The listing builds one solid part. Answer for the finished solid, in the listing's coordinates (mm). Face numbers are marked on the shaded views. A direction names the side the tool comes from. Give positions to 0.01 mm unless a question says otherwise; leave off trailing zeros. Write each loop counter-clockwise with the first axis right and the second up, starting at its lowest first coordinate (ties: lowest second). Pieces come first, ordered by that corner, then holes. Notation, with made-up numbers: (-8.5, 24.25) -> (-3.5, 24.25) arc R17 cw to (-3.5, 31.25) -> close; hole circle Ø4 at (85, 62.25). An arc over 180 degrees is marked (long way). Use CSV: the item, a comma, the result in double quotes. Start each with the question number.
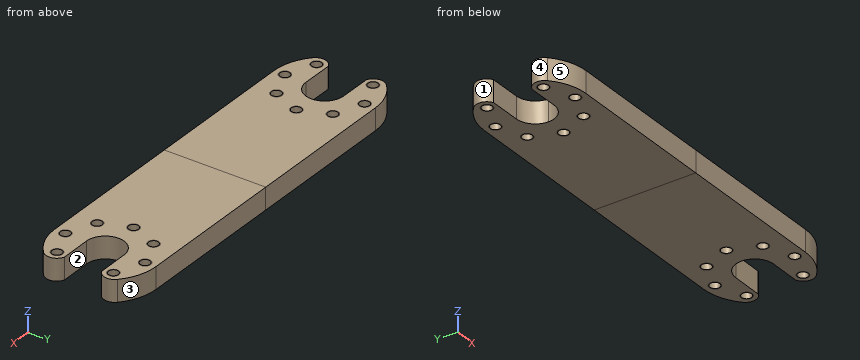
Autodesk Inventor part; units mm, degrees
ref_plane "YZ Plane" through (0, 0, 0) normal (1, 0, 0) x (0, 1, 0)
ref_plane "XZ Plane" through (0, 0, 0) normal (0, 1, 0) x (-1, 0, 0)
ref_plane "XY Plane" through (0, 0, 0) normal (0, 0, 1) x (1, 0, 0)
ref_plane "작업 평면1" through (0, 0, 0) normal (0, 0, 1) x (1, 0, 0)
sketch "스케치1" plane through (0, 0, 0) normal (0, 0, 1) x (1, 0, 0)
  circle A0 centre (-5.2751, -1.5499) radius 1.55
  circle A1 centre (2.5198, 1.6312) radius 1.55
  circle A2 centre (-16.2175, 9.5075) radius 1.55
  circle A3 centre (-13.0363, 1.7126) radius 1.55
  circle A4 centre (-12.955, 17.2687) radius 1.55
  circle A5 centre (-90.374, -1.1049) radius 1.55
  circle A6 centre (-98.1352, 2.1575) radius 1.55
  circle A7 centre (-79.3166, 9.8374) radius 1.55
  circle A8 centre (-82.4977, 17.6323) radius 1.55
  circle A9 centre (-82.579, 2.0762) radius 1.55
  circle A10 centre (-98.0538, 17.7137) radius 1.55
  circle A11 centre (-90.2589, 20.8948) radius 1.55
  circle A12 centre (2.6011, 17.1874) radius 1.55
  circle A13 centre (-5.1601, 20.4498) radius 1.55
  arc A14 (4.3379, -0.782) -> (2.306, 4.4106) centre (2.2903, 1.4106) ccw
  line L0 (2.306, 4.4106) -> (-5.2438, 4.45)
  arc A15 (-5.1915, 14.4499) -> (-5.2438, 4.45) centre (-5.2176, 9.45) ccw
  line L1 (-5.1915, 14.4499) -> (2.3583, 14.4104)
  arc A16 (2.3583, 14.4104) -> (4.4444, 19.5814) centre (2.374, 17.4104) ccw
  arc A17 (4.4444, 19.5814) -> (-5.1444, 23.4498) centre (-5.2176, 9.45) ccw
  line L2 (-5.1444, 23.4498) -> (-90.2432, 23.8948)
  arc A18 (-90.2432, 23.8948) -> (-99.872, 20.1269) centre (-90.3164, 9.8949) ccw
  arc A19 (-99.872, 20.1269) -> (-97.84, 14.9344) centre (-97.8243, 17.9343) ccw
  line L3 (-97.84, 14.9344) -> (-90.2903, 14.8949)
  arc A20 (-90.3426, 4.895) -> (-90.2903, 14.8949) centre (-90.3164, 9.8949) ccw
  line L4 (-90.3426, 4.895) -> (-97.8923, 4.9345)
  arc A21 (-97.8923, 4.9345) -> (-99.9784, -0.2365) centre (-97.908, 1.9345) ccw
  arc A22 (-99.9784, -0.2365) -> (-90.3897, -4.1049) centre (-90.3164, 9.8949) ccw
  line L5 (-90.3897, -4.1049) -> (-90.3897, -4.1065)
  line L6 (-90.3897, -4.1065) -> (-5.2908, -4.5515)
  line L7 (-5.2908, -4.5515) -> (-5.2908, -4.5498)
  arc A23 (-5.2908, -4.5498) -> (4.3379, -0.782) centre (-5.2176, 9.45) ccw
  circle A24 centre (-5.2176, 9.45) radius 1.5
  circle A25 centre (-5.2176, 9.45) radius 5.2
  line L8 (-5.2176, 4.25) -> (6.1788, 4.25)
  line L9 (6.1788, 4.25) -> (6.1788, 14.65)
  line L10 (6.1788, 14.65) -> (-5.2176, 14.65)
  line L11 (-5.2176, 14.65) -> (-5.2176, 4.25)
  circle A26 centre (-12.955, 17.2687) radius 1.35
  circle A27 centre (-16.2175, 9.5075) radius 1.35
  circle A28 centre (-13.0363, 1.7126) radius 1.35
  circle A29 centre (-5.2751, -1.5499) radius 1.35
  circle A30 centre (2.5198, 1.6312) radius 1.35
  circle A31 centre (5.7822, 9.3924) radius 1.35
  circle A32 centre (2.6011, 17.1874) radius 1.35
  circle A33 centre (-5.1601, 20.4498) radius 1.35
  line L12 (-47.6938, 23.6723) -> (-47.8402, -4.329)
  circle A34 centre (-90.374, -1.1049) radius 1.55
  circle A35 centre (-98.1352, 2.1575) radius 1.55
  circle A36 centre (-79.3166, 9.8374) radius 1.55
  circle A37 centre (-82.579, 2.0762) radius 1.55
  circle A38 centre (-82.4977, 17.6323) radius 1.55
  circle A39 centre (-98.0538, 17.7137) radius 1.55
  circle A40 centre (-90.2589, 20.8948) radius 1.55
  arc A41 (-97.8923, 4.9345) -> (-99.9784, -0.2365) centre (-97.908, 1.9345) ccw
  line L13 (-97.8923, 4.9345) -> (-90.3426, 4.895)
  arc A42 (-90.3426, 4.895) -> (-90.2903, 14.8949) centre (-90.3164, 9.8949) ccw
  line L14 (-90.2903, 14.8949) -> (-97.84, 14.9344)
  arc A43 (-99.872, 20.1269) -> (-97.84, 14.9344) centre (-97.8243, 17.9343) ccw
  arc A44 (-90.2432, 23.8948) -> (-99.872, 20.1269) centre (-90.3164, 9.8949) ccw
  line L15 (-90.3897, -4.1065) -> (-90.3897, -4.1049)
  arc A45 (-99.9784, -0.2365) -> (-90.3897, -4.1049) centre (-90.3164, 9.8949) ccw
  circle A46 centre (-90.3164, 9.8949) radius 1.5
  circle A47 centre (-90.3164, 9.8949) radius 5.2
  line L16 (-90.3708, 4.6952) -> (-101.7666, 4.8144)
  line L17 (-101.7666, 4.8144) -> (-101.6578, 15.2138)
  line L18 (-101.6578, 15.2138) -> (-90.2621, 15.0947)
  line L19 (-90.2621, 15.0947) -> (-90.3708, 4.6952)
  circle A48 centre (-82.4977, 17.6323) radius 1.35
  circle A49 centre (-79.3166, 9.8374) radius 1.35
  circle A50 centre (-82.579, 2.0762) radius 1.35
  circle A51 centre (-90.374, -1.1049) radius 1.35
  circle A52 centre (-98.1352, 2.1575) radius 1.35
  circle A53 centre (-101.3163, 9.9525) radius 1.35
  circle A54 centre (-98.0538, 17.7137) radius 1.35
  circle A55 centre (-90.2589, 20.8948) radius 1.35
  point P0 (3.2588, 4.25)
  point P1 (-5.2176, 14.65)
  point P2 (3.5487, 14.65)
  point P3 (-99.0279, 15.1863)
  point P4 (-98.8468, 4.7839)
  dimension "d3" = 0.2
  dimension "d6" = 360
extrude "돌출1" add sketch "스케치1" against normal blind 6 contours A0 | A1 | A2 | A3 | A4 | A5 | A6 | A7 | A8 | A9 | A10 | A11 | A12 | A13 | A23 L6 L12 L2 A17 A16 L10 A25 L8 A14 | L6 A22 A21 L16 A47 L18 A19 A18 L2 L12
properties part number "calf" material "PMMA 플라스틱"
Q1. Section A-A on z = -4.2 is taken. State how many separate pieces and enclosed holes the cut face has, then the cut area to 3 significant figures.
Q2. Straight lines are drawn through the part: L1, parallel to X at y = 9.75, z = -2.05; L2, parallel to X at y = 17.5, z = -4.75; L3, parallel to X at y = 19.75, z = -2.6. For each, find the intervals that lie inside material, in ascending order.
Q3. Flat-ended cylindrical pins translate along their axes: pin 1 Ø4.5 at (x, y) = (-13.04, 1.71) entering from +Z; pin 2 Ø3 at (x, z) = (-9, -1.5) entering from +Y; pin 3 Ø3 at (x, z) = (-43.5, -3.5) entering from -Y; pin 4 Ø3 at (x, z) = (-85.5, -2) entering from +Y. Find the tip coordinate at first contact, or state that the pin passes through.
Q4. The mould has two halves that part along Y. Classify the marked faces 3, 4 and 5: +Y half, -Y half, draft (parallel to the pull), parting line (faces both ways), or undercut.
Q5. Section B-B on y = 13.5 is taken. Give the vertices of the cut face in (x, z).
Q6. For the marked faces 1 and 2, determine the directions among +Z, -Z, +X, -X, +Y, -Y from which every point of the face is accessible in a straight line to the end or side of a thin tool.
Q7. Section C-C on x = -50.5 is taken. Give the vertices of the cut face in (y, z), then the cut area to 3 significant figures.
Output:
1,separate pieces,"1"
1,enclosed holes,"14"
1,area,"2,520 mm²"
2,L1,"-85.12 to -80.66, -77.97 to -17.55, -14.89 to -10.41"
2,L2,"-100.79 to -99.39, -96.72 to -83.84, -81.15 to -14.29, -11.62 to 1.29, 3.91 to 5.37"
2,L3,"-100.21 to -90.97, -89.54 to -6.31, -4.01 to 4.26"
3,pin 1,"z = 0"
3,pin 2,"y = 23.48"
3,pin 3,"y = -4.36"
3,pin 4,"y = 23.88"
4,face 3,"+Y half"
4,face 4,"undercut"
4,face 5,"-Y half"
5,outline,"(-86.57, -6) -> (-8.48, -6) -> (-8.48, 0) -> (-86.57, 0) -> close"
6,face 1,"+Z, -Z, -X"
6,face 2,"+Z, -Z, +X"
7,outline,"(-4.31, -6) -> (23.69, -6) -> (23.69, 0) -> (-4.31, 0) -> close"
7,area,"168 mm²"
